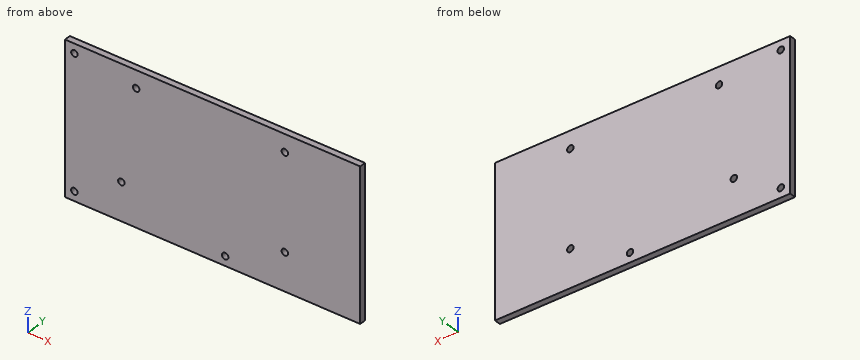
```python
from build123d import *

# Parameters (mm, degrees)
BASE_SKETCH_W                              = 149.225
BASE_SKETCH_H                              = 76.2
BASE_PLATE_DEPTH                           = 3.175
F_4_40_GUIDE_RAIL_HOLES_REACH              = 85.837
F_4_40_HOLE_PATTERN_SKETCH_GUIDE_RAIL_R    = 1.63195
F_4_40_ARDUINO_HOLES_REACH                 = 85.837
F_4_40_HOLE_PATTERN_SKETCH_ARDUINO_HOLES_R = 1.63195


with BuildPart() as part:
    # Base Sketch → Base Plate (new body)
    with BuildSketch(Plane(origin=(0, 0, 0), x_dir=(1, 0, 0), z_dir=(0, 1, 0))):
        Rectangle(BASE_SKETCH_W, BASE_SKETCH_H)
    extrude(amount=BASE_PLATE_DEPTH)

    # 4-40 Hole Pattern Sketch (Guide Rail) → 4-40 Guide Rail Holes (cut, up to next)
    with BuildSketch(Plane(origin=(0, 3.175, 0), x_dir=(1, 0, 0), z_dir=(0, 1, 0)), mode=Mode.PRIVATE) as f_4_40_guide_rail_holes_sk1:
        with Locations(Location((-69.85, 33.3375, 0), (0, 0, 270))):
            Circle(F_4_40_HOLE_PATTERN_SKETCH_GUIDE_RAIL_R)
    f_4_40_guide_rail_holes_tool1 = extrude(f_4_40_guide_rail_holes_sk1.sketch, amount=-F_4_40_GUIDE_RAIL_HOLES_REACH, mode=Mode.PRIVATE) & part.part
    # 4-40 Hole Pattern Sketch (Guide Rail) → 4-40 Guide Rail Holes (cut, up to next)
    with BuildSketch(Plane(origin=(0, 3.175, 0), x_dir=(1, 0, 0), z_dir=(0, 1, 0)), mode=Mode.PRIVATE) as f_4_40_guide_rail_holes_sk2:
        with Locations(Location((-69.85, -33.3375, 0), (0, 0, 270))):
            Circle(F_4_40_HOLE_PATTERN_SKETCH_GUIDE_RAIL_R)
    f_4_40_guide_rail_holes_tool2 = extrude(f_4_40_guide_rail_holes_sk2.sketch, amount=-F_4_40_GUIDE_RAIL_HOLES_REACH, mode=Mode.PRIVATE) & part.part
    # 4-40 Hole Pattern Sketch (Guide Rail) → 4-40 Guide Rail Holes (cut, up to next)
    with BuildSketch(Plane(origin=(0, 3.175, 0), x_dir=(1, 0, 0), z_dir=(0, 1, 0)), mode=Mode.PRIVATE) as f_4_40_guide_rail_holes_sk3:
        with Locations(Location((6.35, 33.3375, 0), (0, 0, 270))):
            Circle(F_4_40_HOLE_PATTERN_SKETCH_GUIDE_RAIL_R)
    f_4_40_guide_rail_holes_tool3 = extrude(f_4_40_guide_rail_holes_sk3.sketch, amount=-F_4_40_GUIDE_RAIL_HOLES_REACH, mode=Mode.PRIVATE) & part.part
    add(f_4_40_guide_rail_holes_tool1.solids().sort_by_distance((-69.85, 3.175, -33.3375))[0], mode=Mode.SUBTRACT)
    add(f_4_40_guide_rail_holes_tool2.solids().sort_by_distance((-69.85, 3.175, 33.3375))[0], mode=Mode.SUBTRACT)
    add(f_4_40_guide_rail_holes_tool3.solids().sort_by_distance((6.35, 3.175, -33.3375))[0], mode=Mode.SUBTRACT)

    # 4-40 Hole Pattern Sketch (Arduino Holes) → 4-40 Arduino Holes (cut, up to next)
    with BuildSketch(Plane(origin=(0, 3.175, 0), x_dir=(1, 0, 0), z_dir=(0, 1, 0)), mode=Mode.PRIVATE) as f_4_40_arduino_holes_sk1:
        with Locations(Location((-46.1137, 19.05, 0), (0, 0, 270))):
            Circle(F_4_40_HOLE_PATTERN_SKETCH_ARDUINO_HOLES_R)
    f_4_40_arduino_holes_tool1 = extrude(f_4_40_arduino_holes_sk1.sketch, amount=-F_4_40_ARDUINO_HOLES_REACH, mode=Mode.PRIVATE) & part.part
    # 4-40 Hole Pattern Sketch (Arduino Holes) → 4-40 Arduino Holes (cut, up to next)
    with BuildSketch(Plane(origin=(0, 3.175, 0), x_dir=(1, 0, 0), z_dir=(0, 1, 0)), mode=Mode.PRIVATE) as f_4_40_arduino_holes_sk2:
        with Locations(Location((-38.6207, -29.2862, 0), (0, 0, 270))):
            Circle(F_4_40_HOLE_PATTERN_SKETCH_ARDUINO_HOLES_R)
    f_4_40_arduino_holes_tool2 = extrude(f_4_40_arduino_holes_sk2.sketch, amount=-F_4_40_ARDUINO_HOLES_REACH, mode=Mode.PRIVATE) & part.part
    # 4-40 Hole Pattern Sketch (Arduino Holes) → 4-40 Arduino Holes (cut, up to next)
    with BuildSketch(Plane(origin=(0, 3.175, 0), x_dir=(1, 0, 0), z_dir=(0, 1, 0)), mode=Mode.PRIVATE) as f_4_40_arduino_holes_sk3:
        with Locations(Location((36.5125, 19.05, 0), (0, 0, 270))):
            Circle(F_4_40_HOLE_PATTERN_SKETCH_ARDUINO_HOLES_R)
    f_4_40_arduino_holes_tool3 = extrude(f_4_40_arduino_holes_sk3.sketch, amount=-F_4_40_ARDUINO_HOLES_REACH, mode=Mode.PRIVATE) & part.part
    # 4-40 Hole Pattern Sketch (Arduino Holes) → 4-40 Arduino Holes (cut, up to next)
    with BuildSketch(Plane(origin=(0, 3.175, 0), x_dir=(1, 0, 0), z_dir=(0, 1, 0)), mode=Mode.PRIVATE) as f_4_40_arduino_holes_sk4:
        with Locations(Location((36.5125, -29.2862, 0), (0, 0, 270))):
            Circle(F_4_40_HOLE_PATTERN_SKETCH_ARDUINO_HOLES_R)
    f_4_40_arduino_holes_tool4 = extrude(f_4_40_arduino_holes_sk4.sketch, amount=-F_4_40_ARDUINO_HOLES_REACH, mode=Mode.PRIVATE) & part.part
    add(f_4_40_arduino_holes_tool1.solids().sort_by_distance((-46.1137, 3.175, -19.05))[0], mode=Mode.SUBTRACT)
    add(f_4_40_arduino_holes_tool2.solids().sort_by_distance((-38.6207, 3.175, 29.2862))[0], mode=Mode.SUBTRACT)
    add(f_4_40_arduino_holes_tool3.solids().sort_by_distance((36.5125, 3.175, -19.05))[0], mode=Mode.SUBTRACT)
    add(f_4_40_arduino_holes_tool4.solids().sort_by_distance((36.5125, 3.175, 29.2862))[0], mode=Mode.SUBTRACT)


solid = part.part
```
Read the model definition and answer for the solid it produces. Units are mm, in the model's axes. Give positions to 0.01 mm unless a question says otherwise; leave off trailing zeros. Order: outer loops, then holes, each group sorted by start corner. A loop starts at its lowest first (then second) coordinate and runs counter-clockwise, first axis right, second up. Notation, with made-up numbers: (-25, 25.5) -> (-20, 25.5) arc R30 ccw to (-20, 57.5) -> close; hole circle Ø7 at (-39.75, 54). An arc over 180 degrees is marked (long way). Write item = value, one per line.
1. A cutting plane is placed at A-A, the plane z = -19.05. Write down the section's boundary in (x, y) (1 decimal).
Numbers:
outline = (-74.6, 0) -> (-47.7, 0) -> (-47.7, 3.2) -> (-74.6, 3.2) -> close; (-44.5, 0) -> (34.9, 0) -> (34.9, 3.2) -> (-44.5, 3.2) -> close; (38.1, 0) -> (74.6, 0) -> (74.6, 3.2) -> (38.1, 3.2) -> close
2. A cutting plane is placed at B-B, the plane x = 6.35. Write down the section's boundary in (y, z) (3 decimals), and give its area (3 significant figures).
Numbers:
outline = (0, -38.1) -> (3.175, -38.1) -> (3.175, -34.969) -> (0, -34.969) -> close; (0, -31.706) -> (3.175, -31.706) -> (3.175, 38.1) -> (0, 38.1) -> close
area = 232 mm²
3. A cutting plane is placed at C-C, the plane x = -69.85. Write down the section's boundary in (y, z) (3 decimals).
Numbers:
outline = (0, -38.1) -> (3.175, -38.1) -> (3.175, -34.969) -> (0, -34.969) -> close; (0, -31.706) -> (3.175, -31.706) -> (3.175, 31.706) -> (0, 31.706) -> close; (0, 34.969) -> (3.175, 34.969) -> (3.175, 38.1) -> (0, 38.1) -> close
4. Given pin 1 (2.5 mm diameter, centred on x = 36.51, z = 29.29, fed in from +Y) (1 decimal), flat-ended and moving along its own axis, determine where the tip first touches the part or whether it passes through.
Numbers:
pin_1 = through
5. Straight lines are drawn through the part: line 1 along X through (y, z) = (1.65, -19.05); line 2 along Z through (x, y) = (-69.85, 1.9); line 3 along Z through (x, y) = (38, 1.15). For each, find the intervals that lie inside material, in ascending order.
Numbers:
line_1 = -74.61 to -47.75, -44.48 to 34.88, 38.14 to 74.61
line_2 = -38.1 to -34.97, -31.71 to 31.71, 34.97 to 38.1
line_3 = -38.1 to -19.72, -18.38 to 28.61, 29.96 to 38.1
